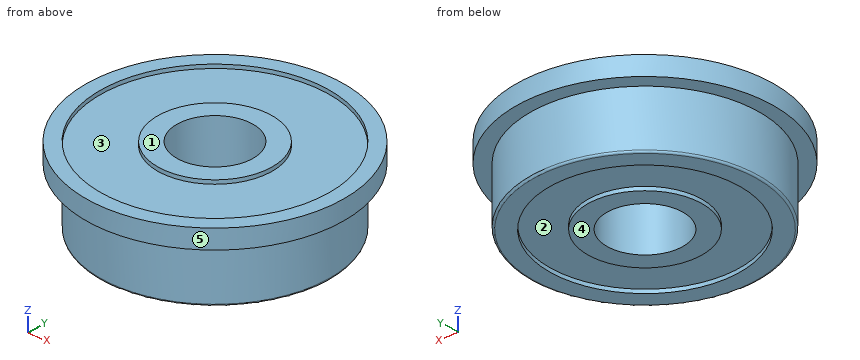
```python
from build123d import *

# Parameters (mm, degrees)
SKETCH_1_R          = 6
EXTRUDE_1_DEPTH     = 4
SKETCH_2_R          = 6.75
EXTRUDE_2_DEPTH     = 1
SKETCH_3_R          = 2
CUT_EXTRUDE_1_DEPTH = 5
SKETCH_4_R          = 5
SKETCH_4_R_2        = 3
CUT_EXTRUDE_2_DEPTH = 0.2
SKETCH_5_R          = 6
SKETCH_5_R_2        = 3
CUT_EXTRUDE_3_DEPTH = 0.2
FILLET_1_R          = 0.1


with BuildPart() as part:
    # 草圖1 → 填料-伸長1 (new body)
    with BuildSketch(Plane.XY):
        Circle(SKETCH_1_R)
    extrude(amount=EXTRUDE_1_DEPTH)

    # 草圖2 → 填料-伸長2 (add)
    with BuildSketch(Plane.XY.offset(4)):
        Circle(SKETCH_2_R)
    extrude(amount=-EXTRUDE_2_DEPTH)

    # 草圖3 → 除料-伸長1 (cut, through all)
    with BuildSketch(Plane(origin=(0, 0, 0), x_dir=(-1, 0, 0), z_dir=(0, 0, -1))):
        Circle(SKETCH_3_R)
    extrude(amount=-CUT_EXTRUDE_1_DEPTH, mode=Mode.SUBTRACT)

    # 草圖4 → 除料-伸長2 (cut)
    with BuildSketch(Plane(origin=(0, 0, 0), x_dir=(-1, 0, 0), z_dir=(0, 0, -1))):
        Circle(SKETCH_4_R)
        Circle(SKETCH_4_R_2, mode=Mode.SUBTRACT)
    extrude(amount=-CUT_EXTRUDE_2_DEPTH, mode=Mode.SUBTRACT)

    # 草圖5 → 除料-伸長3 (cut)
    with BuildSketch(Plane.XY.offset(4)):
        Circle(SKETCH_5_R)
        Circle(SKETCH_5_R_2, mode=Mode.SUBTRACT)
    extrude(amount=-CUT_EXTRUDE_3_DEPTH, mode=Mode.SUBTRACT)

    # 圓角1
    fillet_1_edges = [part.edges().sort_by_distance(p)[0] for p in [
        (-6, 0, 0),
    ]]
    fillet(fillet_1_edges, radius=FILLET_1_R)


solid = part.part
```
Can you work these out from the model? Positions are in its coordinate system, mm. Face numbers are marked on the shaded views. A direction names the side the tool comes from. Give positions to 0.01 mm unless a question says otherwise; leave off trailing zeros. Loops run counter-clockwise (first coordinate to the right, second up) from the corner with the lowest first, then second, coordinate; pieces in that order, holes last. Notation, with made-up numbers: M -5,84 L 10,84 A18 ccw 10,115 Z; hole C 24.5,73.25 d8. An arc over 180 degrees is marked long. Use CSV: the item, a comma, the result in double quotes. Start each with the question number.
1. On a 3-axis mill with a long thin cutter (end or side, diameter ignored), from which of +Z, -Z, +X, -X, +Y, -Y can I reach the whole of each face in a straight line? I mean the marked faces 1 and 2. Say none if no direction works.
2. If I drill on L1, parallel to Y at x = 0, z = 3.95; L2, parallel to Y at x = 0, z = 2.2; L3, parallel to Z at x = -4.5, y = 0.5, over which ranges is the centre line in solid material (lowest first)?
3. For P1, Ø1, axis at x = 3, z = 1, coming from the +Y side, with a flat end and sliding along its axis, tell me the tip position at first contact or that it passes through.
4. Imagine slicing it at C-C, the plane z = 1.25. Write out the boundary of the cut face in (x, y).
5. Imagine slicing it at D-D, the plane z = 3.6. Write out the boundary of the cut face in (x, y), plus the area to 3 significant figures.
6. If we mould it in two halves opening along X, with no side actions, what happens to the marked faces 3, 4 and 5? For each: released by +X, released by -X, zero draft, split by the parting line, or undercut.
Response values:
1,face 1,"+Z, +X, -X, +Y, -Y"
1,face 2,"-Z"
2,L1,"-6.75 to -6, -3 to -2, 2 to 3, 6 to 6.75"
2,L2,"-6 to -2, 2 to 6"
2,L3,"0.2 to 3.8"
3,P1,"y = 5.45"
4,outline,"C 0,0 d12; hole C 0,0 d4"
5,outline,"C 0,0 d13.5; hole C 0,0 d4"
5,area,"131 mm^2"
6,face 3,"undercut"
6,face 4,"zero draft"
6,face 5,"split by the parting line"
